Geometry check sheet. Reference: drawing and pictorial views, mm from the part's lowest x, y, z. A direction names the side the tool comes from. Round coordinates to 2 decimals unless told otherwise and drop trailing zeros. Order: outer loops, then holes, each group sorted by start corner. A loop starts at its lowest first (then second) coordinate and runs counter-clockwise, first axis right, second up.
(1) Material ranges on line 1 along Z through (x, y) = (6.9, 12.7); line 2 along Y through (x, z) = (8.5, 5.08); line 3 along Z through (x, y) = (3.2, 63.5), recorded low to high.
(2) Sectioned sample at D-D (z = 27). Record the boundary of the cut face in (x, y) (1 decimal), plus the area to 3 significant figures.
(3) Go/stop test with flat-tipped pins: pin 1 (4 mm diameter, centred on y = 62, z = 53.5, fed in from -X); pin 2 (1.5 mm diameter, centred on y = 61.5, z = 36.5, fed in from -X); pin 3 (2.5 mm diameter, centred on y = 63.5, z = 5.08, fed in from +X); pin 4 (8.5 mm diameter, centred on y = 65, z = 6.5, fed in from -X). Record where each tip stops, or that it passes through.
(4) Sectioned sample at A-A (y = 12.7). Give the number of separate pieces and of enclosed holes in the cut face.
(5) Set-up check for the marked faces 1, 2 and 3: record each of +Z, -Z, +X, -X, +Y, -Y from which the full face is reachable in a straight line by a thin tool's end or side.
(6) Sectioned sample at B-B (z = 5.08). Record the boundary of the cut face in (x, y) (1 decimal).
(7) Sectioned sample at C-C (y = 22). Record the boundary of the cut face in (x, z) (1 decimal), plus the area to 3 significant figures.
(8) Release check for a two-part mould opening along Z. For the marked faces 4 and 5 record: +Z half, -Z half, draft (parallel to the pull), parting line (faces both ways), or undercut.
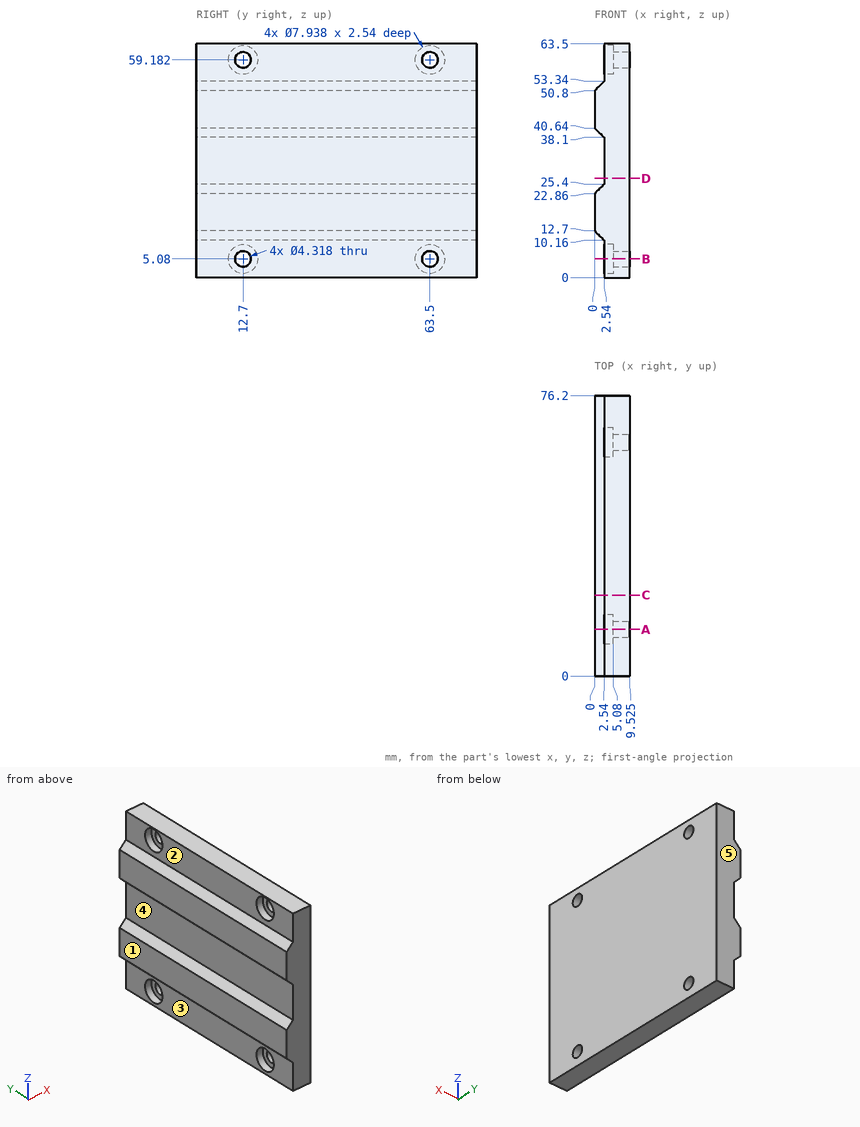
Answer below:
1. line 1: z = 0 to 2.92, 7.24 to 57.02, 61.34 to 63.5
1. line 2: y = 0 to 10.54, 14.86 to 61.34, 65.66 to 76.2
1. line 3: z = 0 to 1.11, 9.05 to 55.21, 63.15 to 63.5
2. outline: (2.5, 0) - (9.5, 0) - (9.5, 76.2) - (2.5, 76.2) - close
2. area: 532 mm2
3. pin 1: stops at x = 0.7
3. pin 2: stops at x = 2.54
3. pin 3: passes through
3. pin 4: stops at x = 1.95
4. separate pieces: 3
4. enclosed holes: 0
5. face 1: +Z, -Z, -X, +Y, -Y
5. face 2: +Z, -X, +Y, -Y
5. face 3: -Z, -X, +Y, -Y
6. outline: (2.5, 0) - (9.5, 0) - (9.5, 10.5) - (5.1, 10.5) - (5.1, 8.7) - (2.5, 8.7) - close; (2.5, 16.7) - (5.1, 16.7) - (5.1, 14.9) - (9.5, 14.9) - (9.5, 61.3) - (5.1, 61.3) - (5.1, 59.5) - (2.5, 59.5) - close; (2.5, 67.5) - (5.1, 67.5) - (5.1, 65.7) - (9.5, 65.7) - (9.5, 76.2) - (2.5, 76.2) - close
7. outline: (0, 12.7) - (2.5, 10.2) - (2.5, 0) - (9.5, 0) - (9.5, 63.5) - (2.5, 63.5) - (2.5, 53.3) - (0, 50.8) - (0, 40.6) - (2.5, 38.1) - (2.5, 25.4) - (0, 22.9) - close
7. area: 508 mm2
8. face 4: undercut
8. face 5: draft
